Verification items for the finished model (mm, model axes). Round coordinates to 2 decimals unless told otherwise and drop trailing zeros. Order: outer loops, then holes, each group sorted by start corner. A loop starts at its lowest first (then second) coordinate and runs counter-clockwise, first axis right, second up. Notation, with made-up numbers: M 86.5,72.25 L 124.5,72.25 A6 ccw 124.5,82.25 Z; hole C 85,-5 d10. An arc over 180 degrees is marked long. Use one line per item in the form item = value. Start each with the question number.
Item 1: Thickness scan on probe 1 along Y at (x, z) = (-62, 42); probe 2 along X at (y, z) = (60, 38.6); probe 3 along X at (y, z) = (1, 41). Record the ranges inside material, lowest first. Write a range as [from, to].
Item 2: Cross-section at A-A on x = 99.5. Enter the section's corners in (y, z).
Item 3: Release check for a two-part mould opening along Y. For faces 1 (the flat face through (56.996, 81.597, 40.958)), 2 (the flat face through (-81.597, 56.996, 40.958)), 3 (the flat face through (-40, -42, 38)) record: +Y half, -Y half, draft (parallel to the pull), parting line (faces both ways), or undercut.
Item 4: Cross-section at C-C on y = 104. Enter the section's corners in (x, z), then the cut area to 3 significant figures.
Item 5: Cross-section at D-D on x = 13. Enter the section's corners in (y, z), then the cut area to 3 significant figures.
Item 6: Cross-section at B-B on y = -3.5. Enter the section's corners in (x, z), then the cut area to 4 significant figures.
Item 7: Go/stop test with flat-tipped pins: pin 1 Ø3 at (y, z) = (40.5, 40) entering from -X; pin 2 Ø1 at (x, z) = (-28, 41) entering from -Y. Record where each tip stops, or that it passes through.
Autodesk Inventor part; units mm, degrees
ref_plane "YZ Plane" through (0, 0, 0) normal (1, 0, 0) x (0, 1, 0)
ref_plane "XZ Plane" through (0, 0, 0) normal (0, 1, 0) x (-1, 0, 0)
ref_plane "XY Plane" through (0, 0, 0) normal (0, 0, 1) x (1, 0, 0)
ref_plane "РабПлоскость1" through (-64.3467, 78.4889, 38) normal (0, 0, 1) x (-0.7071, -0.7071, 0)
sketch "Эскиз1" plane through (-64.3467, 78.4889, 38) normal (0, 0, 1) x (-0.7071, -0.7071, 0)
  circle A0 centre (10, 101) radius 135
  line L0 (35, 205) -> (35, 199)
  line L1 (35, 199) -> (20, 199)
  line L2 (20, 199) -> (20, 205)
  line L3 (20, 205) -> (35, 205)
  line L4 (-15, 205) -> (0, 205)
  line L5 (0, 205) -> (0, 199)
  line L6 (0, 199) -> (-15, 199)
  line L7 (-15, 199) -> (-15, 205)
  line L8 (114, 76) -> (108, 76)
  line L9 (108, 76) -> (108, 91)
  line L10 (108, 91) -> (114, 91)
  line L11 (114, 91) -> (114, 76)
  line L12 (114, 126) -> (114, 111)
  line L13 (114, 111) -> (108, 111)
  line L14 (108, 111) -> (108, 126)
  line L15 (108, 126) -> (114, 126)
  line L16 (-15, -3) -> (-15, 3)
  line L17 (-15, 3) -> (0, 3)
  line L18 (0, 3) -> (0, -3)
  line L19 (0, -3) -> (-15, -3)
  line L20 (35, -3) -> (20, -3)
  line L21 (20, -3) -> (20, 3)
  line L22 (20, 3) -> (35, 3)
  line L23 (35, 3) -> (35, -3)
  line L24 (-88, 111) -> (-94, 111)
  line L25 (-94, 111) -> (-94, 126)
  line L26 (-94, 126) -> (-88, 126)
  line L27 (-88, 126) -> (-88, 111)
  line L28 (-94, 91) -> (-88, 91)
  line L29 (-88, 91) -> (-88, 76)
  line L30 (-88, 76) -> (-94, 76)
  line L31 (-94, 76) -> (-94, 91)
  circle A1 centre (10, 101) radius 50
  circle A2 centre (10, 101) radius 135
  circle A3 centre (81.4178, 29.5822) radius 26.5
  circle A4 centre (-61.4178, 29.5822) radius 26.5
  circle A5 centre (-61.4178, 172.4178) radius 26.5
  circle A6 centre (81.4178, 172.4178) radius 26.5
  point P0 (10, 101)
extrude "Выдавливание1" add sketch "Эскиз1" along normal blind 6
properties part number "Диск_верхний_В5" material "По умолчанию1"
Output values:
q1.probe_1 = [-119.92, -85.08], [-76.59, 76.59], [85.08, 119.92]
q1.probe_2 = [-120.93, -87.08], [-78.59, 78.59], [87.08, 120.93]
q1.probe_3 = [-135, -127.48], [-74.52, -49.99], [49.99, 74.52], [127.48, 135]
q2.outline = M -91.24,38 L -26.46,38 L -26.46,44 L -91.24,44 Z; M 26.46,38 L 91.24,38 L 91.24,44 L 26.46,44 Z
q3.face_1 = undercut
q3.face_2 = undercut
q3.face_3 = draft
q4.outline = M -86.08,38 L -26.33,38 L -26.33,44 L -86.08,44 Z; M 26.33,38 L 86.08,38 L 86.08,44 L 26.33,44 Z
q4.area = 717 mm2
q5.outline = M -134.37,38 L -124.09,38 L -124.09,44 L -134.37,44 Z; M -77.91,38 L -48.28,38 L -48.28,44 L -77.91,44 Z; M 48.28,38 L 77.91,38 L 77.91,44 L 48.28,44 Z; M 124.09,38 L 134.37,38 L 134.37,44 L 124.09,44 Z
q5.area = 479 mm2
q6.outline = M -134.95,38 L -127.27,38 L -127.27,44 L -134.95,44 Z; M -74.73,38 L -49.88,38 L -49.88,44 L -74.73,44 Z; M 49.88,38 L 74.73,38 L 74.73,44 L 49.88,44 Z; M 127.27,38 L 134.95,38 L 134.95,44 L 127.27,44 Z
q6.area = 390.5 mm2
q7.pin_1 = -129.24
q7.pin_2 = -132.17
